Work out the finished part from the listing and answer in its coordinate system (mm). A direction names the side the tool comes from. Give positions to 0.01 mm unless a question says otherwise; leave off trailing zeros. Loops run counter-clockwise (first coordinate to the right, second up) from the corner with the lowest first, then second, coordinate; pieces in that order, holes last. Notation, with made-up numbers: M 42.25,-22.75 L 93.25,-22.75 A22 ccw 93.25,11.25 Z; hole C 41,-15.5 d3. An arc over 180 degrees is marked long. Answer in a Markdown table with one row per item. Add a question column.
Autodesk Inventor part; units mm, degrees
ref_plane "YZ Plane" through (0, 0, 0) normal (1, 0, 0) x (0, 1, 0)
ref_plane "XZ Plane" through (0, 0, 0) normal (0, 1, 0) x (-1, 0, 0)
ref_plane "XY Plane" through (0, 0, 0) normal (0, 0, 1) x (1, 0, 0)
sketch "Sketch1" plane through (0, 0, 0) normal (0, 1, 0) x (-1, 0, 0)
  line L0 (0, 0) -> (0, -40) construction
  line L1 (-1.65, 0) -> (-1.65, -40)
  line L2 (1.65, -40) -> (1.65, 0)
  arc A0 (1.65, 0) -> (-1.65, 0) centre (0, 0) ccw
  arc A1 (-1.65, -40) -> (1.65, -40) centre (0, -40) ccw
  line L3 (-5, 10) -> (7.65, 10)
  line L4 (7.65, 10) -> (7.65, -50)
  line L5 (7.65, -50) -> (-5, -50)
  line L6 (-5, -50) -> (-5, 10)
  circle A2 centre (0, -40) radius 5
  circle A3 centre (0, 0) radius 5
  point P0 (0, -20)
  dimension "d0" = 3.3
  dimension "d1" = 40
  dimension "d2" = 10
  dimension "d3" = 10
  dimension "d4" = 10
  dimension "d5" = 10
  dimension "d6" = 6
extrude "Extrusion1" add sketch "Sketch1" along normal blind 10 contours L1 A3 L2 A0 | L1 A2 L6 A3 | L1 A1 L2 A2 | L6 L3 L4 L5 A2 L2 A3 picked at (-2.0178, -2.9645) picked at (-2.0178, -37.0355)
ref_plane "Work Plane1" through (0, 0, 0) normal (1, 0, 0) x (0, 0, -1)
properties part number "Rail"
(1) Consider line 1 along X through (y, z) = (3.5, -38.5); line 2 along Z through (x, y) = (0.5, 6.5). Determine where each line is inside the solid, lowest interval first. Write a range as from..to.
(2) The mould has two halves that part along X. Classify faces 3 (the face through (-0.04, 4.93, -41.65)), 4 (the face through (-7.65, 5, -20)), 5 (the face through (5, 5, -20)): pulls with the +X half, pulls with the -X half, needs draft (parallel to the pull), parting line crosses it, or undercut.
(3) Section A-A, the plane x = 0 is taken. Determine the outline of the cut face in (y, z), and give its area (3 significant figures).
(4) Section C-C, the plane y = 3 is taken. Determine the outline of the cut face in (x, z), and give its area (3 significant figures).
(5) Section B-B, the plane z = -9 is taken. Determine the outline of the cut face in (x, y).
(6) Which of the six approach directions +Z, -Z, +X, -X, +Y, -Y give full straight-line access (tool end or side, diameter ignored) to faces 1 (the face through (1.65, 5, -20)), 2 (the face through (-3, 10, -20))?
Numbers:
| question | item | result |
|---|---|---|
| 1 | line 1 | x = -7.65..-1.65, 1.65..5 |
| 1 | line 2 | z = -50..-41.57, 1.57..10 |
| 2 | face 3 | undercut |
| 2 | face 4 | pulls with the -X half |
| 2 | face 5 | pulls with the +X half |
| 3 | outline | M 0,-50 L 10,-50 L 10,-41.65 L 0,-41.65 Z; M 0,1.65 L 10,1.65 L 10,10 L 0,10 Z |
| 3 | area | 167 mm² |
| 4 | outline | M -7.65,-50 L 5,-50 L 5,10 L -7.65,10 Z; hole M -1.65,-40 A1.65 ccw 1.65,-40 L 1.65,0 A1.65 ccw -1.65,0 Z |
| 4 | area | 618 mm² |
| 5 | outline | M -7.65,0 L -1.65,0 L -1.65,10 L -7.65,10 Z; M 1.65,0 L 5,0 L 5,10 L 1.65,10 Z |
| 6 | face 1 | +Y, -Y |
| 6 | face 2 | +Z, -Z, +X, -X, +Y |
